Check sheet for the modelled part. Datum: model origin and axes. Units: mm. Face numbers are marked on the shaded views. A direction names the side the tool comes from. Round coordinates to 2 decimals unless told otherwise and drop trailing zeros. Order: outer loops, then holes, each group sorted by start corner. A loop starts at its lowest first (then second) coordinate and runs counter-clockwise, first axis right, second up.
```python
from build123d import *

# Parameters (mm, degrees)
SKETCH1_W                          = 76.2
SKETCH1_H                          = 12.7
BOSS_EXTRUDE1_DEPTH                = 117.55
F_2_5MM_DOWEL_HOLE2_D              = 2.5
SKETCH13_W                         = 56
SKETCH13_H                         = 76.2
BOSS_EXTRUDE3_DEPTH                = 35.45
SKETCH11_R                         = 3.75
CUT_EXTRUDE3_DEPTH                 = 24.5
SKETCH14_R                         = 1.905
CUT_EXTRUDE4_DEPTH                 = 24.65
TAP_DRILL_FOR_M2_5X0_45_TAP1_D     = 2.05
TAP_DRILL_FOR_M2_5X0_45_TAP1_DEPTH = 8.3
TAP_DRILL_FOR_M2_5X0_45_TAP1_TIP   = 0.615882135


with BuildPart() as part:
    # Sketch1 → Boss-Extrude1 (new body)
    with BuildSketch(Plane(origin=(0, 0, 0), x_dir=(0, 0, -1), z_dir=(1, 0, 0))):
        with Locations((0, 6.903854155)):
            Rectangle(SKETCH1_W, SKETCH1_H)
    extrude(amount=BOSS_EXTRUDE1_DEPTH)

    # Ø2.5mm Dowel Hole2 (through all)
    with Locations(Plane(origin=(0, 13.253854155, 0), x_dir=(1, 0, 0), z_dir=(0, 1, 0))):
        with Locations((12, 0), (34, 0), (23, -11), (23, 11)):
            Hole(F_2_5MM_DOWEL_HOLE2_D / 2)

    # Sketch13 → Boss-Extrude3 (add)
    with BuildSketch(Plane(origin=(0, 13.253854155, 0), x_dir=(1, 0, 0), z_dir=(0, 1, 0))):
        with Locations((89.55, 0)):
            Rectangle(SKETCH13_W, SKETCH13_H)
    extrude(amount=BOSS_EXTRUDE3_DEPTH)

    # Sketch11 → Cut-Extrude3 (cut)
    with BuildSketch(Plane(origin=(0, 0.553854155, 0), x_dir=(1, 0, 0), z_dir=(0, 1, 0))):
        with Locations((104.375, 13.4747)):
            Circle(SKETCH11_R)
        with Locations((74.695, 13.4747)):
            Circle(SKETCH11_R)
    cut_extrude3 = extrude(amount=CUT_EXTRUDE3_DEPTH, mode=Mode.SUBTRACT)

    # Sketch14 → Cut-Extrude4 (cut, through all)
    with BuildSketch(Plane.XZ.offset(-25.053854155)):
        with Locations((104.375, -13.4747)):
            Circle(SKETCH14_R)
        with Locations((74.695, -13.4747)):
            Circle(SKETCH14_R)
    cut_extrude4 = extrude(amount=-CUT_EXTRUDE4_DEPTH, mode=Mode.SUBTRACT)

    # Mirror2: Cut-Extrude3, Cut-Extrude4 across plane
    add(cut_extrude3.mirror(Plane.XY), mode=Mode.SUBTRACT)
    add(cut_extrude4.mirror(Plane.XY), mode=Mode.SUBTRACT)

    # Tap Drill for M2.5x0.45 Tap1
    with Locations(Plane.ZY):
        with Locations((-12.7, 6.903854155), (12.7, 6.903854155)):
            Hole(TAP_DRILL_FOR_M2_5X0_45_TAP1_D / 2, depth=TAP_DRILL_FOR_M2_5X0_45_TAP1_DEPTH)
            with Locations((0, 0, -(TAP_DRILL_FOR_M2_5X0_45_TAP1_DEPTH + TAP_DRILL_FOR_M2_5X0_45_TAP1_TIP / 2))):  # 118° drill point
                Cone(0, TAP_DRILL_FOR_M2_5X0_45_TAP1_D / 2, TAP_DRILL_FOR_M2_5X0_45_TAP1_TIP, mode=Mode.SUBTRACT)


solid = part.part
```
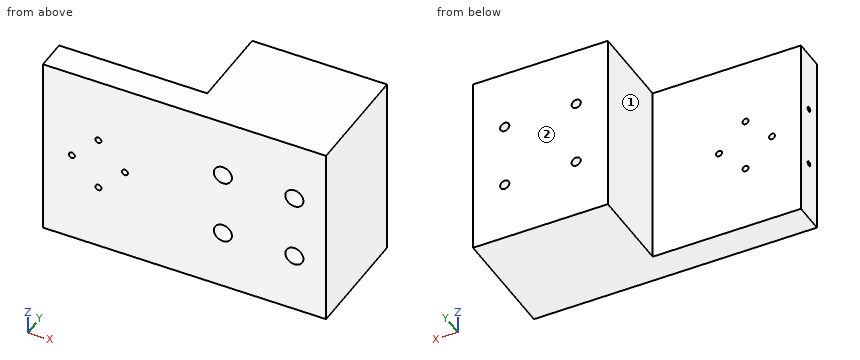
Item 1: Go/stop test with flat-tipped pins: P1, Ø12, axis at x = 104.38, z = 13.47, coming from the +Y side; P2, Ø2, axis at x = 75, z = -15, coming from the -Y side; P3, Ø1, axis at y = 29, z = -21, coming from the -X side. Record where each tip stops, or that it passes through.
Answer:
P1: stops at y = 48.7
P2: stops at y = 25.05
P3: stops at x = 61.55
Item 2: Scan lines: line 1 along Z through (x, y) = (73, 21.5); line 2 along X through (y, z) = (19, 16); line 3 along Z through (x, y) = (34, 3). Record each from-to range of solid material in increasing order.
Answer:
line 1: z = -38.1 to -16.82, -10.13 to 10.13, 16.82 to 38.1
line 2: x = 61.55 to 71.92, 77.47 to 101.6, 107.15 to 117.55
line 3: z = -38.1 to -1.25, 1.25 to 38.1
Item 3: Sectioned sample at A-A (x = 34). Record the cut outline in (y, z).
Answer:
outline: (0.55, -38.1) - (13.25, -38.1) - (13.25, -1.25) - (0.55, -1.25) - close; (0.55, 1.25) - (13.25, 1.25) - (13.25, 38.1) - (0.55, 38.1) - close
Item 4: Sectioned sample at C-C (y = 21). Record the cut outline in (x, z) (3 decimals), and give its area (3 significant figures).
Answer:
outline: (61.55, -38.1) - (117.55, -38.1) - (117.55, 38.1) - (61.55, 38.1) - close; hole circle Ø7.5 at (74.695, -13.475); hole circle Ø7.5 at (74.695, 13.475); hole circle Ø7.5 at (104.375, -13.475); hole circle Ø7.5 at (104.375, 13.475)
area: 4,090 mm2
Item 5: Sectioned sample at B-B (z = 0). Record the cut outline in (x, y), and give its area (3 significant figures).
Answer:
outline: (0, 0.55) - (10.75, 0.55) - (10.75, 13.25) - (0, 13.25) - close; (13.25, 0.55) - (32.75, 0.55) - (32.75, 13.25) - (13.25, 13.25) - close; (35.25, 0.55) - (117.55, 0.55) - (117.55, 48.7) - (61.55, 48.7) - (61.55, 13.25) - (35.25, 13.25) - close
area: 3,410 mm2
Item 6: Access from +Z, -Z, +X, -X, +Y, -Y to the whole of each face (thin tool, end or side, straight path). Record for the marked faces 1 and 2.
Answer:
face 1: +Z, -Z, -X, +Y
face 2: +Z, -Z, +X, -X, +Y
Item 7: Sectioned sample at D-D (x = 74). Record the cut outline in (y, z), and give its area (3 significant figures).
Answer:
outline: (0.55, -38.1) - (48.7, -38.1) - (48.7, -15.25) - (25.05, -15.25) - (25.05, -17.16) - (0.55, -17.16) - close; (0.55, -9.79) - (25.05, -9.79) - (25.05, -11.7) - (48.7, -11.7) - (48.7, 11.7) - (25.05, 11.7) - (25.05, 9.79) - (0.55, 9.79) - close; (0.55, 17.16) - (25.05, 17.16) - (25.05, 15.25) - (48.7, 15.25) - (48.7, 38.1) - (0.55, 38.1) - close
area: 3,140 mm2
